```python
from build123d import *

# Parameters (mm, degrees)
F1_DEPTH = 4
F2_COUNT = 4
F4_DEPTH = 5


with BuildPart() as f1:
    # F0 (on Top) → F1 (new body)
    with BuildSketch(Plane.XY):
        with BuildLine():
            Line((-11.3897752017, 0), (0, 0))
            Line((0, 0), (0, 11.2630287185))
            Line((0, 11.2630287185), (-5.4190037772, 11.2630287185))
            Line((-5.4190037772, 11.2630287185), (-5.4190037772, 11.0505186021))
            Line((-5.4190037772, 11.0505186021), (-8.6066536605, 16.7882870883))
            ThreePointArc((-8.6066536605, 16.7882870883), (-6.5795750519, 28.2187096113), (-13.0392942344, 37.8642077748))
            ThreePointArc((-13.0392942344, 37.8642077748), (-24.1128062403, 39.6994920993), (-30.5027211192, 30.4712785919))
            ThreePointArc((-30.5027211192, 30.4712785919), (-28.9257647374, 18.8694362404), (-20.024523139, 11.2630287185))
            Line((-20.024523139, 11.2630287185), (-20.024523139, 0))
            Line((-20.024523139, 0), (-11.3897752017, 0))
        make_face()
    extrude(amount=F1_DEPTH)

    # F2: F1 ×4 about axis
    f2_axis = Axis((0, 0, 2), (0, 0, -1))


with BuildPart() as f1_1:
    add(f1.part)
    for i in range(1, F2_COUNT):
        add(f1.part.rotate(f2_axis, i * 360 / F2_COUNT))

    # F3 (on face) → F4 (cut)
    with BuildSketch(Plane.XY.offset(4)):
        with BuildLine():
            ThreePointArc((0, 6.5), (-4.5961940777, -4.5961940777), (6.5, 0))
            ThreePointArc((6.5, 0), (4.5961940777, 4.5961940777), (0, 6.5))
        make_face()
    extrude(amount=-F4_DEPTH, mode=Mode.SUBTRACT)


solid = f1_1.part
```
Geometry check sheet. Reference: the model listing, model coordinates, mm. A direction names the side the tool comes from. Round coordinates to 2 decimals unless told otherwise and drop trailing zeros. Order: outer loops, then holes, each group sorted by start corner. A loop starts at its lowest first (then second) coordinate and runs counter-clockwise, first axis right, second up. Notation, with made-up numbers: (-9, -11) -> (25, -11) arc R13 cw to (25, 10) -> close; hole circle Ø5 at (-12, 39). An arc over 180 degrees is marked (long way). Return JSON: item names as keys, results as strings. Group by question number.
Q1. Material ranges on probe 1 along X at (y, z) = (-0.5, 1.75); probe 2 along Y at (x, z) = (-5.5, 2.65); probe 3 along X at (y, z) = (-12, 1.8), recorded low to high. Write a range as from..to.
Q2. Tool access check on faces 5 (the flat face through (0, -16, 2)), 6 (the flat face through (20.025, -6, 2)), 7 (the flat face through (-11.263, -3, 2)), 8 (the flat face through (6, 20.025, 2)), 9 (the cylindrical face through (-28.056, -6.546, 1.972)). Record the directions out of +Z, -Z, +X, -X, +Y, -Y that give a thin tool (end or side, any length) a straight path to the whole face; none if there is none.
Q3. Gauge pin test, flat ends, axial feed: pin 1 (11.5 mm diameter, centred on x = 0, y = 0, fed in from +Z); pin 2 (1.2 mm diameter, centred on x = 7, z = 2, fed in from +Y); pin 3 (1 mm diameter, centred on y = 30, z = 1.5, fed in from -X); pin 4 (2 mm diameter, centred on y = -4, z = 1.5, fed in from -X). Record the tip position at first contact, or that the pin passes through.
Q4. Section check B-B, the plane y = -2.5. Record the boundary of the cut face in (x, z).
Q5. Release check for a two-part mould opening along Y. For faces 1 (the flat face through (-16, 0, 2)), 2 (the flat face through (0, 16, 2)), 3 (the cylindrical face through (-23.96, 39.763, 1.972)), 4 (the cylindrical face through (-19.017, -29.005, 1.972)) record: released by +Y, released by -Y, zero draft, split by the parting line, or undercut.
Q6. Section check C-C, the plane x = -18.5. Record the boundary of the cut face in (y, z), plus the area to 3 significant figures.
Numbers:
{
 "1": {"probe 1": "-11.26..-6.48, 6.48..20.02", "probe 2": "-20.02..-3.46, 3.46..11.2", "probe 3": "-37.09..0, 5.95..21.77"},
 "2": {"face 5": "+Z, -Z, -Y", "face 6": "+Z, -Z, +X", "face 7": "+Z, -Z, -X", "face 8": "+Z, -Z, +Y", "face 9": "+Z, -Z"},
 "3": {"pin 1": "through", "pin 2": "y = 20.02", "pin 3": "x = -30.7", "pin 4": "x = -11.26"},
 "4": {"outline": "(-11.26, 0) -> (-6, 0) -> (-6, 4) -> (-11.26, 4) -> close; (6, 0) -> (20.02, 0) -> (20.02, 4) -> (6, 4) -> close"},
 "5": {"face 1": "undercut", "face 2": "zero draft", "face 3": "released by +Y", "face 4": "released by -Y"},
 "6": {"outline": "(-28.72, 0) -> (-7.68, 0) -> (-7.68, 4) -> (-28.72, 4) -> close; (0, 0) -> (40.42, 0) -> (40.42, 4) -> (0, 4) -> close", "area": "246 mm^2"}
}
